Check sheet for the modelled part. Datum: model origin and axes. Units: mm. Face numbers are marked on the shaded views. A direction names the side the tool comes from. Coordinates: 2 decimals unless noted, no trailing zeros. Loops run counter-clockwise (first coordinate to the right, second up) from the corner with the lowest first, then second, coordinate; pieces in that order, holes last. Notation, with made-up numbers: M 77,-31 L 97,-31 A29 cw 97,-10 Z; hole C 24.25,45 d5. An arc over 180 degrees is marked long. Use CSV: the item, a comma, the result in double quotes. Start each with the question number.
(1) Section check A-A on x = 0. Record the cut outline in (y, z).
(2) Section check D-D on y = -27.5. Record the cut outline in (x, z), and give its area (3 significant figures).
(3) Section check B-B on y = -19. Record the cut outline in (x, z), and give its area (3 significant figures).
(4) Set-up check for the marked faces 4, 5 and 6: record each of +Z, -Z, +X, -X, +Y, -Y from which the full face is reachable in a straight line by a thin tool's end or side.
(5) Scan lines: line 1 (Y direction, x = 0, z = -10.5); line 2 (Z direction, x = -2, y = -15.5); line 3 (X direction, y = -27.5, z = 16.25). Record each from-to range of solid material in increasing order.
(6) Draft check along Z on the marked faces 1, 2 and 3. Enter one of: pulls with the +Z half, pulls with the -Z half, needs draft (parallel to the pull), parting line crosses it, or undercut.
(7) Section check C-C on z = -12. Record the cut outline in (x, y).
(8) Go/stop test with flat-tipped pins: pin 1 Ø5.5 at (y, z) = (-26, -12.5) entering from -X; pin 2 Ø3 at (x, z) = (1, 18.5) entering from +Y; pin 3 Ø6 at (y, z) = (-5, -9.5) entering from +X; pin 4 Ø1.5 at (x, z) = (-6.5, 18.5) entering from -Y. Record where each tip stops, or that it passes through.
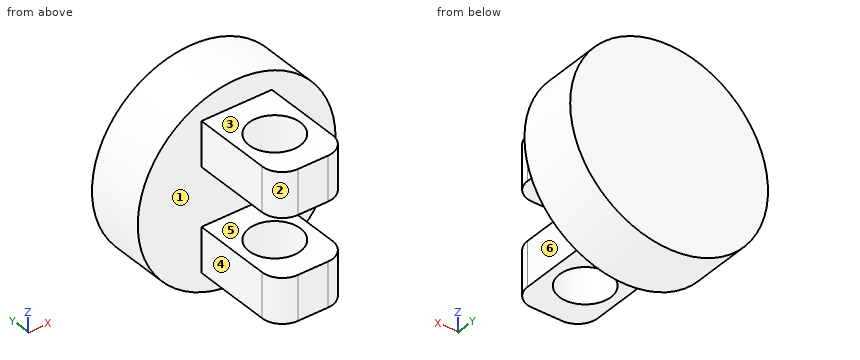
from build123d import *

# Parameters (mm, degrees)
F0_R     = 25
F1_DEPTH = 15
F2_W     = 17.784364
F2_H     = 37.209642
F3_DEPTH = 25
F6_D     = 13
F4_W     = 17.784364
F4_H     = 14.687386
F7_DEPTH = 25
F8_R     = 5.08


with BuildPart() as f1:
    # F0 (on Front) → F1 (new body)
    with BuildSketch(Plane.XZ):
        Circle(F0_R)
    extrude(amount=F1_DEPTH)

    # F2 (on face) → F3 (join)
    with BuildSketch(Plane.XZ.offset(15)):
        Rectangle(F2_W, F2_H)
    extrude(amount=F3_DEPTH)

    # F6 (through all)
    with Locations(Plane(origin=(0, 0, -18.604821), x_dir=(1, 0, 0), z_dir=(0, 0, -1))):
        with Locations((0, 27.5)):
            Hole(F6_D / 2)

    # F4 (on face) → F7 (cut)
    with BuildSketch(Plane.XZ.offset(40)):
        Rectangle(F4_W, F4_H)
    extrude(amount=-F7_DEPTH, mode=Mode.SUBTRACT)

    # F8
    f8_edges = [f1.edges().sort_by_distance(p)[0] for p in [
        (8.892182, -40, -12.974257),
        (8.892182, -40, 12.974257),
        (-8.892182, -40, 12.974257),
        (-8.892182, -40, -12.974257),
    ]]
    fillet(f8_edges, radius=F8_R)


solid = f1.part
Outcome:
1,outline,"M -40,-18.6 L -34,-18.6 L -34,-7.34 L -40,-7.34 Z; M -40,7.34 L -34,7.34 L -34,18.6 L -40,18.6 Z; M -21,-18.6 L -15,-18.6 L -15,-25 L 0,-25 L 0,25 L -15,25 L -15,18.6 L -21,18.6 L -21,7.34 L -15,7.34 L -15,-7.34 L -21,-7.34 Z"
2,outline,"M -8.89,-18.6 L -6.5,-18.6 L -6.5,-7.34 L -8.89,-7.34 Z; M -8.89,7.34 L -6.5,7.34 L -6.5,18.6 L -8.89,18.6 Z; M 6.5,-18.6 L 8.89,-18.6 L 8.89,-7.34 L 6.5,-7.34 Z; M 6.5,7.34 L 8.89,7.34 L 8.89,18.6 L 6.5,18.6 Z"
2,area,"108 mm²"
3,outline,"M -8.89,-18.6 L 8.89,-18.6 L 8.89,-7.34 L -8.89,-7.34 Z; M -8.89,7.34 L 8.89,7.34 L 8.89,18.6 L -8.89,18.6 Z"
3,area,"401 mm²"
4,face 4,"+Z, -Z, -X, -Y"
4,face 5,"+X, -X, -Y"
4,face 6,"+Z, -Z, +X, -Y"
5,line 1,"y = -40 to -34, -21 to 0"
5,line 2,"z = -18.6 to -7.34, 7.34 to 18.6"
5,line 3,"x = -8.89 to -6.5, 6.5 to 8.89"
6,face 1,"undercut"
6,face 2,"needs draft"
6,face 3,"pulls with the +Z half"
7,outline,"M -21.93,-15 L -8.89,-15 L -8.89,-34.92 A5.08 ccw -3.81,-40 L 3.81,-40 A5.08 ccw 8.89,-34.92 L 8.89,-15 L 21.93,-15 L 21.93,0 L -21.93,0 Z; hole C 0,-27.5 d13"
8,pin 1,"stops at x = -8.89"
8,pin 2,"stops at y = 0"
8,pin 3,"stops at x = 24.14"
8,pin 4,"stops at y = -39.62"
